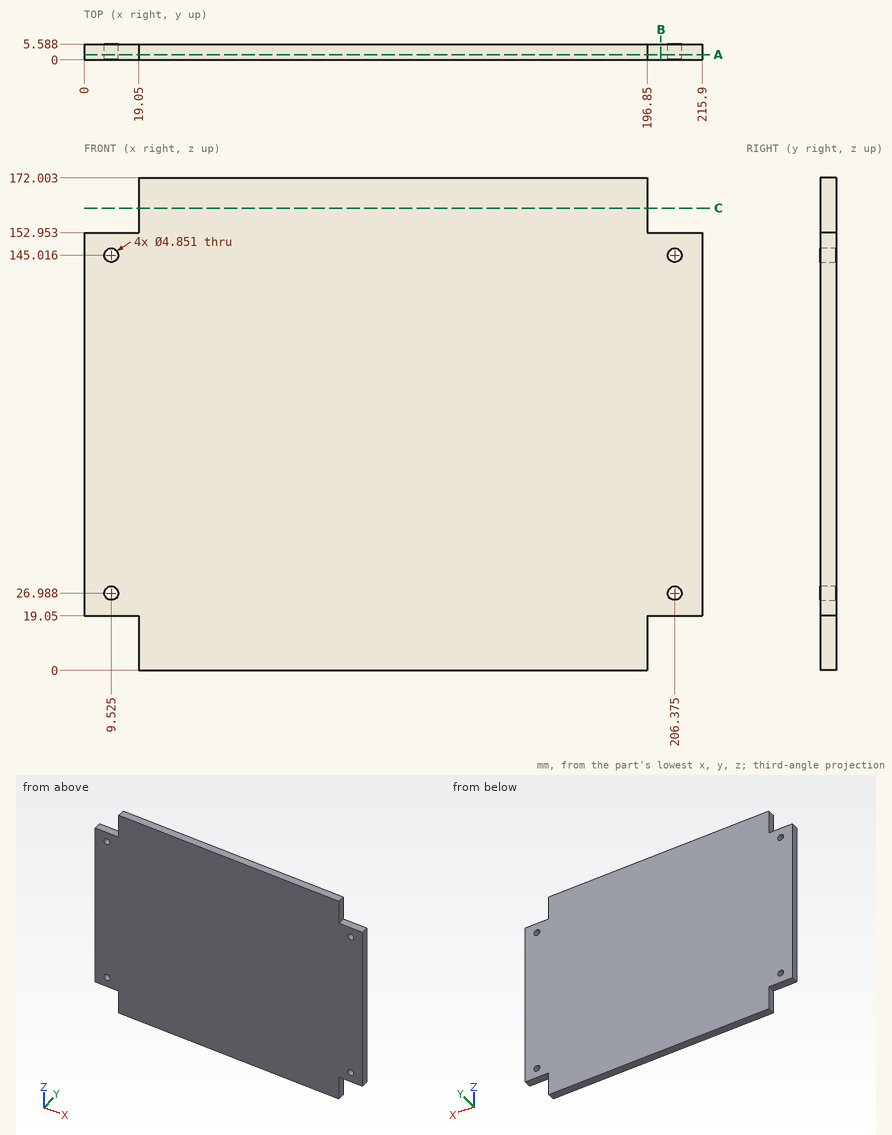
Geometry: see drawing. Coordinates: mm, zero at the bounding-box minimum. Round coordinates to 2 decimals unless told otherwise and drop trailing zeros. Loops run counter-clockwise (first coordinate to the right, second up) from the corner with the lowest first, then second, coordinate; pieces in that order, holes last. Notation, with made-up numbers: M 63.5,29 L 119.5,29 A8 ccw 119.5,40 Z; hole C 6,24.5 d7. An arc over 180 degrees is marked long. Use a Markdown table: item, result. Add a question column.
1. Ray query, line 1 along X through (y, z) = (1.5, 25) (1 decimal); line 2 along X through (y, z) = (1.2, 14); line 3 along X through (y, z) = (2.15, 29). Return the intervals inside material, ascending. Write a range as [from, to].
2. Cut plane B-B, the plane x = 201.5. Output: boundary loops of the cut face in (y, z).
3. Cut plane A-A, the plane y = 1.9. State how many separate pieces and enclosed holes the cut face has, and give its area (3 significant figures).
4. Contact query for flat-ended pins moving along their axis: pin 1 (1.7 mm diameter, centred on y = 3, z = 12.5, fed in from -X); pin 2 (4 mm diameter, centred on x = 9.53, z = 26.99, fed in from -Y); pin 3 (6 mm diameter, centred on x = 30, z = 92.5, fed in from -Y); pin 4 (3 mm diameter, centred on x = 6.5, y = 4, fed in from +Z). Output: stop coordinate, or through.
5. Cut plane C-C, the plane z = 161.5. Output: boundary loops of the cut face in (x, y).
Solution:
| question | item | result |
|---|---|---|
| 1 | line 1 | x = [0, 8.1], [10.9, 205], [207.8, 215.9] |
| 1 | line 2 | x = [19.05, 196.85] |
| 1 | line 3 | x = [0, 8.17], [10.88, 205.02], [207.73, 215.9] |
| 2 | outline | M 0,19.05 L 5.59,19.05 L 5.59,152.95 L 0,152.95 Z |
| 3 | separate pieces | 1 |
| 3 | enclosed holes | 4 |
| 3 | area | 35,600 mm2 |
| 4 | pin 1 | stops at x = 19.05 |
| 4 | pin 2 | passes through |
| 4 | pin 3 | stops at y = 0 |
| 4 | pin 4 | stops at z = 152.95 |
| 5 | outline | M 19.05,0 L 196.85,0 L 196.85,5.59 L 19.05,5.59 Z |
